Design review of the part built by this model. Coordinates are the model's own, in mm. Coordinates: 2 decimals unless noted, no trailing zeros. Loops run counter-clockwise (first coordinate to the right, second up) from the corner with the lowest first, then second, coordinate; pieces in that order, holes last. Notation, with made-up numbers: (23.25, 59) -> (62.25, 59) arc R12 cw to (62.25, 74) -> close; hole circle Ø9 at (-19, 6.5). An arc over 180 degrees is marked (long way). Use one line per item in the form item = value. Start each with the question number.
1. Consider section A-A (x = -101.75). State the section outline as (y, z) points (3 decimals).
2. Consider section B-B (y = -206). State the section outline as (x, z) points (3 decimals), then the cut area to 3 significant figures.
3. Wall thickness on line 1 (Y direction, x = -112.5, z = 15); line 2 (Z direction, x = -95.75, y = -176.5) (3 decimals); line 3 (Y direction, x = -104.5, z = 112.5): over which ranges is each line inside the solid? List them lowest first. Write a range as from..to.
4. Consider section C-C (z = 143). State the section outline as (x, y) points.
5. For pin 1 (1 mm diameter, centred on x = -108, y = -174, fed in from -Z); pin 2 (9.5 mm diameter, centred on x = -106.5, y = -203.5, fed in from +Z) (3 decimals); pin 3 (6 mm diameter, centred on x = -99.5, y = 11.5, fed in from +Z); pin 4 (5.5 mm diameter, centred on x = -101, z = 72, fed in from -Y), all flat-tipped, find the tip position at first contact; note any pin that passes through.
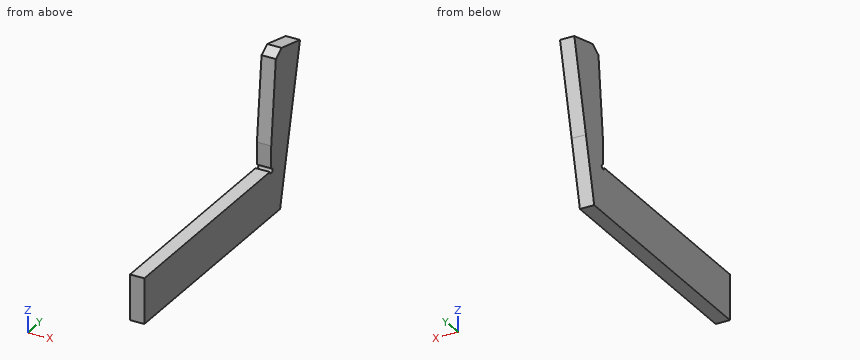
from build123d import *

# Parameters (mm, degrees)
BOSS_EXTRUDE1_DEPTH = 19.05
BOSS_EXTRUDE2_DEPTH = 19.05
CHAMFER1_SIZE       = 12.7
CHAMFER1_SIZE2      = 11.325028866


with BuildPart() as part:
    # Sketch2 → Boss-Extrude1 (new body)
    with BuildSketch(Plane(origin=(-113.788766336, 0, 0), x_dir=(0, 0, -1), z_dir=(1, 0, 0))):
        with BuildLine():
            Line((0, 20.824633003), (-83.828599938, 40.306941911))
            Line((-83.828599938, 40.306941911), (-93.196193981, 0))
            Line((-93.196193981, 0), (-63.5, 0))
            ThreePointArc((-63.5, 0), (-58.07993597, 2.24506403), (-60.325, -3.175))
            Line((-60.325, -3.175), (-60.325, -298.45))
            Line((-60.325, -298.45), (0, -298.45))
            Line((0, -298.45), (0, 20.824633003))
        make_face()
    extrude(amount=BOSS_EXTRUDE1_DEPTH)

    # Sketch3 → Boss-Extrude2 (add, through all)
    with BuildSketch(Plane.ZY.offset(113.788766336)):
        Polygon((83.828599938, 40.306941911), (201.08567571, 67.558244849), (214.022912031, 11.891823944), (93.196193981, 0), align=None)
    extrude(amount=-BOSS_EXTRUDE2_DEPTH)

    # Chamfer1
    chamfer1_edges = [part.edges().sort_by_distance(p)[0] for p in [
        (-104.263766336, 11.891823944, 214.022912031),
    ]]
    chamfer1_side = [part.faces().sort_by_distance(p)[0] for p in [
        (-104.263766336, 39.725034397, 207.554293871),
    ]]
    chamfer(chamfer1_edges, length=CHAMFER1_SIZE, length2=CHAMFER1_SIZE2, reference=chamfer1_side[0])


solid = part.part
Geometry check:
q1.outline = (-298.45, 0) -> (20.825, 0) -> (67.558, 201.086) -> (24.262, 211.148) -> (10.783, 202.752) -> (0, 93.196) -> (0, 63.5) arc R3.175 cw (long way) to (-3.175, 60.325) -> (-298.45, 60.325) -> close
q2.outline = (-113.789, 0) -> (-94.739, 0) -> (-94.739, 60.325) -> (-113.789, 60.325) -> close
q2.area = 1,150 mm²
q3.line_1 = -298.45..24.31
q3.line_2 = 0..60.325
q3.line_3 = 1.9..46.97
q4.outline = (-113.79, 4.9) -> (-94.74, 4.9) -> (-94.74, 54.06) -> (-113.79, 54.06) -> close
q5.pin_1 = 0
q5.pin_2 = 60.325
q5.pin_3 = 205.07
q5.pin_4 = 0
